from build123d import *

# Parameters (mm, degrees)
F1_DEPTH = 30.1625
F2_W     = 23.8125
F2_H     = 15.875
F3_DEPTH = 6.35
F4_R     = 2.921
F5_DEPTH = 6.35


# Not quite as in the source:
# - a feature names something its author has since deleted; it is built from what else it names


with BuildPart() as f1:
    # F0 (on Top) → F1 (new body)
    with BuildSketch(Plane.XY):
        Polygon((-40.48125, 0), (0, 0), (40.48125, 0), (49.3395, -43.65625), (49.3395, -69.1896), (55.6895, -69.1896), (74.7395, -69.1896), (74.7395, -62.8396), (55.6895, -62.8396), (55.6895, -43.0185116827), (45.6721801749, 6.35), (0, 6.35), (-45.6721801749, 6.35), (-55.6895, -43.0185116827), (-55.6895, -62.8396), (-74.7395, -62.8396), (-74.7395, -69.1896), (-55.6895, -69.1896), (-49.3395, -69.1896), (-49.3395, -43.65625), align=None)
    extrude(amount=F1_DEPTH)

    # F2 (on face) → F3 (cut, through all)
    with BuildSketch(Plane.XZ):
        with Locations((-19.05, 14.2875)):
            Rectangle(F2_W, F2_H)
        with Locations((19.05, 14.2875)):
            Rectangle(F2_W, F2_H)
    extrude(amount=-F3_DEPTH, mode=Mode.SUBTRACT)

    # F4 (on face) → F5 (cut, through all)
    with BuildSketch(Plane(origin=(0, -62.8396, 0), x_dir=(-1, 0, 0), z_dir=(0, 1, 0))):
        with Locations((65.2145, 15.08125)):
            Circle(F4_R)
        with Locations((-65.2145, 15.08125)):
            Circle(F4_R)
    extrude(amount=-F5_DEPTH, mode=Mode.SUBTRACT)


solid = f1.part
Part model, mm, in its own coordinate system. A direction names the side the tool comes from. Round coordinates to 2 decimals unless told otherwise and drop trailing zeros. Write each loop counter-clockwise with the first axis right and the second up, starting at its lowest first coordinate (ties: lowest second). Pieces come first, ordered by that corner, then holes. Notation, with made-up numbers: M 70.5,-19.75 L 97.5,-19.75 A20 cw 97.5,1.25 Z; hole C 44,9.5 d3. An arc over 180 degrees is marked long. Return JSON: item names as keys, results as strings. Group by question number.
(1) Pin check, flat tips, straight feed: pin 1 Ø5 at (y, z) = (4.5, 13) entering from +X; pin 2 Ø7.5 at (y, z) = (-57, 9) entering from +X; pin 3 Ø1.5 at (x, z) = (-35.5, 4) entering from -Y; pin 4 Ø3.5 at (x, z) = (65.21, 15.08) entering from -Y. Stop position of each tip, or through.
(2) Two-plate mould, pull along Z, no slides. Class faces 1 (the face through (5, 2, 30.162)), 2 (the face through (-50.61, -17.99, 14.87)), 3 (the face through (19, 3, 22.225)): +Z half, -Z half, draft (parallel to the pull), parting line (faces both ways), or undercut.
(3) Saw through at B-B on z = 26.5. Write the cut outline in (x, y), then the cut area to 3 significant figures.
(4) Saw through at C-C on y = -27. Write the cut outline in (x, z).
(5) Drill centre lines: probe 1 along X at (y, z) = (-50.5, 20.5); probe 2 along Y at (x, z) = (-59, 19); probe 3 along Y at (x, z) = (2, 16). Where is each one in solid material? Low to high.
(6) Which spindle directions (+Z, -Z, +X, -X, +Y, -Y) get a long thin tool onto all of the face, cutting with end or side? Do faces 4 (the face through (49.34, -56, 15)), 5 (the face through (-7.144, 3, 14)), 6 (the face through (-65, -62.84, 12)), 7 (the face through (55.69, -53, 15)). Say none if no direction does.
Returned:
{
 "1": {"pin 1": "x = 46.55", "pin 2": "x = 55.69", "pin 3": "y = 0", "pin 4": "through"},
 "2": {"face 1": "+Z half", "face 2": "draft", "face 3": "undercut"},
 "3": {"outline": "M -74.74,-69.19 L -49.34,-69.19 L -49.34,-43.66 L -40.48,0 L 40.48,0 L 49.34,-43.66 L 49.34,-69.19 L 74.74,-69.19 L 74.74,-62.84 L 55.69,-62.84 L 55.69,-43.02 L 45.67,6.35 L -45.67,6.35 L -55.69,-43.02 L -55.69,-62.84 L -74.74,-62.84 Z", "area": "1,720 mm²"},
 "4": {"outline": "M -52.44,0 L -45.96,0 L -45.96,30.16 L -52.44,30.16 Z; M 45.96,0 L 52.44,0 L 52.44,30.16 L 45.96,30.16 Z"},
 "5": {"probe 1": "-55.69 to -49.34, 49.34 to 55.69", "probe 2": "-69.19 to -62.84", "probe 3": "0 to 6.35"},
 "6": {"face 4": "+Z, -Z, -Y", "face 5": "+Y, -Y", "face 6": "+Z, -Z, -X, +Y", "face 7": "+Z, -Z, +X, +Y"}
}
